from build123d import *

# Parameters (mm, degrees)
F1_DEPTH = 25
F3_DEPTH = 25
F4_DEPTH = 50.001
F5_W     = 0.25
F5_H     = 7.4
F5_W_2   = 7.4
F5_H_2   = 0.25
F6_DEPTH = 25.001


with BuildPart() as f1:
    # F0 (on Top) → F1 (new body)
    with BuildSketch(Plane.XY):
        with BuildLine():
            ThreePointArc((30, 4.5), (27.656854, 10.156854), (22, 12.5))
            Line((22, 12.5), (-22, 12.5))
            ThreePointArc((-22, 12.5), (-27.656854, 10.156854), (-30, 4.5))
            Line((-30, 4.5), (-30, -4.5))
            ThreePointArc((-30, -4.5), (-27.656854, -10.156854), (-22, -12.5))
            Line((-22, -12.5), (22, -12.5))
            ThreePointArc((22, -12.5), (27.656854, -10.156854), (30, -4.5))
            Line((30, -4.5), (30, 4.5))
        make_face()
    extrude(amount=F1_DEPTH)

    # F2 (on face) → F3 (join)
    with BuildSketch(Plane.XY.offset(25)):
        with BuildLine():
            ThreePointArc((22, 1.5), (21.12132, 3.62132), (19, 4.5))
            Line((19, 4.5), (-19, 4.5))
            ThreePointArc((-19, 4.5), (-21.12132, 3.62132), (-22, 1.5))
            Line((-22, 1.5), (-22, -1.5))
            ThreePointArc((-22, -1.5), (-21.12132, -3.62132), (-19, -4.5))
            Line((-19, -4.5), (19, -4.5))
            ThreePointArc((19, -4.5), (21.12132, -3.62132), (22, -1.5))
            Line((22, -1.5), (22, 1.5))
        make_face()
    extrude(amount=F3_DEPTH)

    # F3_face (on face) → F4 (cut, through all)
    with BuildSketch(Plane.XY.offset(50)):
        with BuildLine():
            ThreePointArc((22, 1.5), (21.12132, 3.62132), (19, 4.5))
            Line((19, 4.5), (-19, 4.5))
            ThreePointArc((-19, 4.5), (-21.12132, 3.62132), (-22, 1.5))
            Line((-22, 1.5), (-22, -1.5))
            ThreePointArc((-22, -1.5), (-21.12132, -3.62132), (-19, -4.5))
            Line((-19, -4.5), (19, -4.5))
            ThreePointArc((19, -4.5), (21.12132, -3.62132), (22, -1.5))
            Line((22, -1.5), (22, 1.5))
        make_face()
    extrude(amount=-F4_DEPTH, mode=Mode.SUBTRACT)

    # F5 (on face) → F6 (cut, through all)
    with BuildSketch(Plane.XY.offset(25)):
        with Locations((-19.475, 8.8)):
            Rectangle(F5_W, F5_H)
        with Locations((19.475, 8.8)):
            Rectangle(F5_W, F5_H)
        with Locations((-19.475, -8.8)):
            Rectangle(F5_W, F5_H)
        with Locations((19.475, -8.8)):
            Rectangle(F5_W, F5_H)
        with Locations((26.3, -1.975)):
            Rectangle(F5_W_2, F5_H_2)
        with Locations((26.3, 1.975)):
            Rectangle(F5_W_2, F5_H_2)
        with Locations((-26.3, 1.975)):
            Rectangle(F5_W_2, F5_H_2)
        with Locations((-26.3, -1.975)):
            Rectangle(F5_W_2, F5_H_2)
        with Locations((0, -8.8)):
            Rectangle(F5_W, F5_H)
        with Locations((0, 8.8)):
            Rectangle(F5_W, F5_H)
    extrude(amount=-F6_DEPTH, mode=Mode.SUBTRACT)


solid = f1.part
Geometry: final body of the model. Coordinates: model frame, mm. A direction names the side the tool comes from. Give positions to 0.01 mm unless a question says otherwise; leave off trailing zeros. Order: outer loops, then holes, each group sorted by start corner. A loop starts at its lowest first (then second) coordinate and runs counter-clockwise, first axis right, second up. Notation, with made-up numbers: (2.5, 5.5) - (8.5, 5.5) arc R15 cw to (8.5, 9.5) - close; hole circle Ø9 at (-36.75, -12). An arc over 180 degrees is marked (long way). Use CSV: the item, a comma, the result in double quotes.
1. Contact query for flat-ended pins moving along their axis: pin 1 (3.5 mm diameter, centred on x = 25.5, z = 11.5, fed in from +Y); pin 2 (6 mm diameter, centred on x = 27, z = 16, fed in from +Y); pin 3 (6 mm diameter, centred on x = -26.5, z = 13.5, fed in from +Y). Output: stop coordinate, or through.
Answers below:
pin 1,"y = 12.31"
pin 2,"y = 12.25"
pin 3,"y = 12.36"
2. Section query C-C (y = 6.5). Output: boundary loops of the cut face in (x, z) (3 decimals), plus the area to 3 significant figures.
Answers below:
outline,"(-29.746, 0) - (-19.6, 0) - (-19.6, 25) - (-29.746, 25) - close; (-19.35, 0) - (-0.125, 0) - (-0.125, 25) - (-19.35, 25) - close; (0.125, 0) - (19.35, 0) - (19.35, 25) - (0.125, 25) - close; (19.6, 0) - (29.746, 0) - (29.746, 25) - (19.6, 25) - close"
area,"1,470 mm2"
3. Section query A-A (x = -11). Output: boundary loops of the cut face in (y, z), plus the area to 3 significant figures.
Answers below:
outline,"(-12.5, 0) - (-4.5, 0) - (-4.5, 25) - (-12.5, 25) - close; (4.5, 0) - (12.5, 0) - (12.5, 25) - (4.5, 25) - close"
area,"400 mm2"
4. Access query for faces 1 (the face through (-10, -12.5, 12)), 2 (the face through (0.125, 9, 13)), 3 (the face through (21.1, -3.64, 12.67)), 4 (the face through (30, 0, 12)), 5 (the face through (19.6, -9, 13)). Directions: +Z, -Z, +X, -X, +Y, -Y. A direction counts if a zero-diameter tool reaches every point of the face in a straight line with its end or side. Return the directions, or none.
Answers below:
face 1,"+Z, -Z, +X, -X, -Y"
face 2,"+Z, -Z, +Y"
face 3,"+Z, -Z"
face 4,"+Z, -Z, +X, +Y, -Y"
face 5,"+Z, -Z, -Y"
5. Section query B-B (y = 0.25). Output: boundary loops of the cut face in (x, z), plus the area to 3 significant figures.
Answers below:
outline,"(-30, 0) - (-22, 0) - (-22, 25) - (-30, 25) - close; (22, 0) - (30, 0) - (30, 25) - (22, 25) - close"
area,"400 mm2"
6. Section query D-D (y = 11.25). Output: boundary loops of the cut face in (x, z) (3 decimals).
Answers below:
outline,"(-26.294, 0) - (-19.6, 0) - (-19.6, 25) - (-26.294, 25) - close; (-19.35, 0) - (-0.125, 0) - (-0.125, 25) - (-19.35, 25) - close; (0.125, 0) - (19.35, 0) - (19.35, 25) - (0.125, 25) - close; (19.6, 0) - (26.294, 0) - (26.294, 25) - (19.6, 25) - close"
7. Mould query, pull axis Y, two halves, no side actions, for faces 6 (the face through (19.6, 9, 13)), 7 (the face through (10, -12.5, 12)), 8 (the face through (-27.594, 10.219, 12.325)), 9 (the face through (-26, 2.1, 13)). Classes: +Y half, -Y half, draft (parallel to the pull), parting line (faces both ways), or undercut.
Answers below:
face 6,"draft"
face 7,"-Y half"
face 8,"+Y half"
face 9,"undercut"
8. Material intervals for line 1 along Y through (x, z) = (-19, 2); line 2 along X through (y, z) = (-7.75, 11.75) (3 decimals); line 3 along X through (y, z) = (6, 12.25) (3 decimals), sorted ascending. Write a range as from..to.
Answers below:
line 1,"-12.5..-4.5, 4.5..12.5"
line 2,"-29.31..-19.6, -19.35..-0.125, 0.125..19.35, 19.6..29.31"
line 3,"-29.858..-19.6, -19.35..-0.125, 0.125..19.35, 19.6..29.858"
